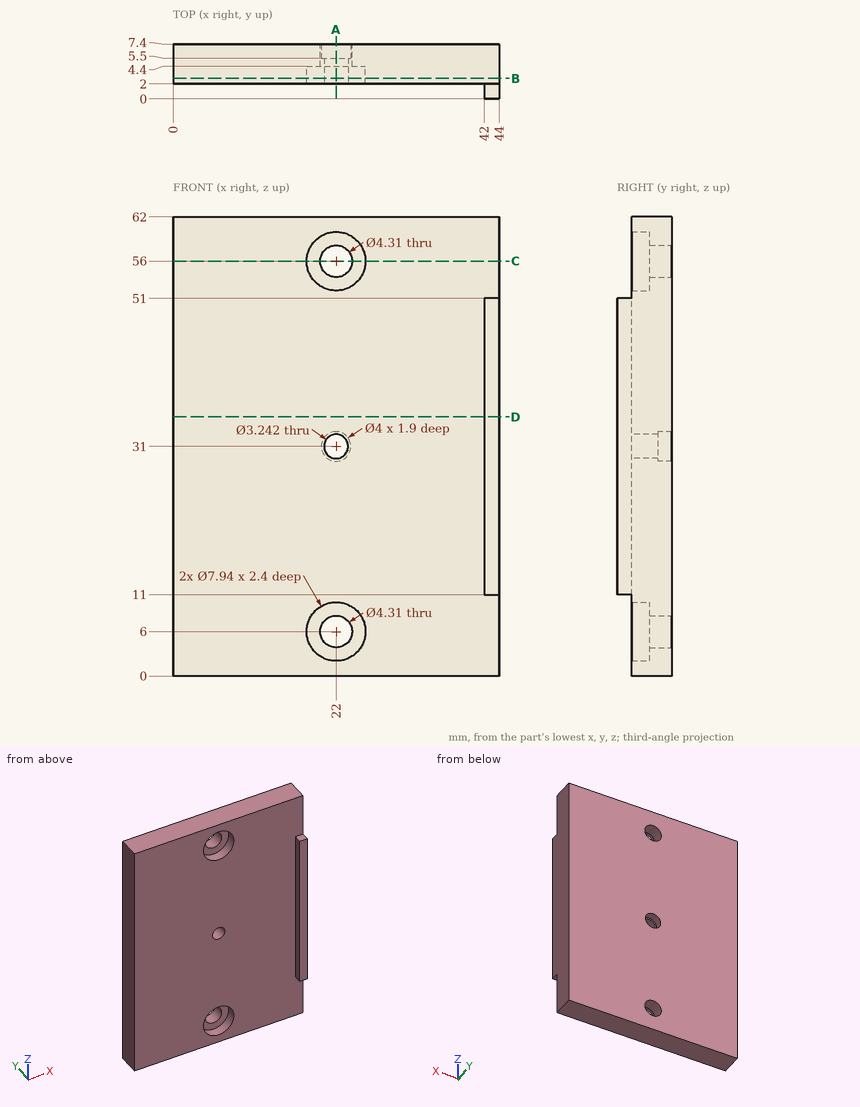
Source: three-view drawing plus pictorial views. Frame: mm from the lowest corner of the part. Give positions to 0.01 mm unless a question says otherwise; leave off trailing zeros. Order: outer loops, then holes, each group sorted by start corner. A loop starts at its lowest first (then second) coordinate and runs counter-clockwise, first axis right, second up. Notation, with made-up numbers: (46.25, -9.75) - (71.25, -9.75) arc R33 ccw to (71.25, 18.25) - close; hole circle Ø6 at (32, -3). An arc over 180 degrees is marked (long way). Put each result on its own line as item: value.
Item 1: Contact query for flat-ended pins moving along their axis: pin 1 (0.6 mm diameter, centred on x = 43.5, y = 1, fed in from +Z); pin 2 (5 mm diameter, centred on x = 22, z = 6, fed in from -Y); pin 3 (2.5 mm diameter, centred on x = 22, z = 6, fed in from -Y); pin 4 (8.5 mm diameter, centred on x = 23.5, z = 7, fed in from -Y). Output: stop coordinate, or through.
Found:
pin 1: stops at z = 51
pin 2: stops at y = 4.4
pin 3: passes through
pin 4: stops at y = 2
Item 2: Section query D-D, the plane z = 35. Return loops of the section in (x, y), then the cut area to 3 significant figures.
Found:
outline: (0, 2) - (42, 2) - (42, 0) - (44, 0) - (44, 7.4) - (0, 7.4) - close
area: 242 mm^2
Item 3: Section query A-A, the plane x = 22. Return loops of the section in (y, z) (3 decimals).
Found:
outline: (2, 0) - (7.4, 0) - (7.4, 3.845) - (4.4, 3.845) - (4.4, 2.03) - (2, 2.03) - close; (2, 9.97) - (4.4, 9.97) - (4.4, 8.155) - (7.4, 8.155) - (7.4, 29) - (5.5, 29) - (5.5, 29.379) - (2, 29.379) - close; (2, 32.621) - (5.5, 32.621) - (5.5, 33) - (7.4, 33) - (7.4, 53.845) - (4.4, 53.845) - (4.4, 52.03) - (2, 52.03) - close; (2, 59.97) - (4.4, 59.97) - (4.4, 58.155) - (7.4, 58.155) - (7.4, 62) - (2, 62) - close
Item 4: Section query B-B, the plane y = 2.75. Return loops of the section in (x, z), then the cut area to 3 significant figures.
Found:
outline: (0, 0) - (44, 0) - (44, 62) - (0, 62) - close; hole circle Ø7.94 at (22, 6); hole circle Ø7.94 at (22, 56); hole circle Ø3.24 at (22, 31)
area: 2,620 mm^2
Item 5: Ray query, L1, parallel to Z at x = 22, y = 2.65; L2, parallel to X at y = 3.75, z = 6; L3, parallel to X at y = 6.7, z = 31. Return the intervals inside material, ascending. Write a range as from..to.
Found:
L1: z = 0..2.03, 9.97..29.38, 32.62..52.03, 59.97..62
L2: x = 0..18.03, 25.97..44
L3: x = 0..20, 24..44
Item 6: Section query C-C, the plane z = 56. Return loops of the section in (x, y) (3 decimals), then the cut area to 3 significant figures.
Found:
outline: (0, 2) - (18.03, 2) - (18.03, 4.4) - (19.845, 4.4) - (19.845, 7.4) - (0, 7.4) - close; (24.155, 4.4) - (25.97, 4.4) - (25.97, 2) - (44, 2) - (44, 7.4) - (24.155, 7.4) - close
area: 206 mm^2
